Can you work these out from the model? Positions are in its coordinate system, mm. Face numbers are marked on the shaded views. Coordinates: 2 decimals unless noted, no trailing zeros. Order: outer loops, then holes, each group sorted by start corner. A loop starts at its lowest first (then second) coordinate and runs counter-clockwise, first axis right, second up. Notation, with made-up numbers: (8.5, 43.5) -> (31.5, 43.5) arc R8 cw to (31.5, 57.5) -> close; hole circle Ø9 at (62, -34.75). An arc over 180 degrees is marked (long way). Use a Markdown table: item, result. Add a question column.
1. We'd pull the mould along X, two halves only. Please class the marked faces 1 and 2: pulls with the +X half, pulls with the -X half, needs draft (parallel to the pull), parting line crosses it, or undercut.
2. Suppose I cut it at C-C, the plane z = 5.5. List the corners of the cut face in (x, y) for me.
3. Suppose I cut it at A-A, the plane y = 0. List the corners of the cut face in (x, z) for me.
4. If I drill on line 1 along Y through (x, z) = (-1.15, 4.5); line 2 along Y through (x, z) = (0.5, 1.25); line 3 along X through (y, z) = (-0.85, 2), over which ranges is the centre line in solid material (lowest first)? Write a range as from..to.
5. For pin 1 Ø1 at (x, z) = (-1.5, 3) entering from -Y; pin 2 Ø2.5 at (y, z) = (-0.5, 3.5) entering from -X; pin 3 Ø1.5 at (y, z) = (-1.5, 1.5) entering from +X, each with a flat end and sliding along its axis, tell me the tip position at first contact or that it passes through.
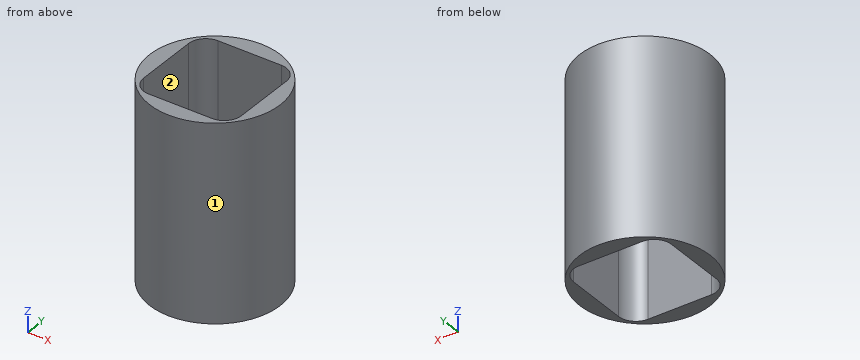
```python
from build123d import *

# Parameters (mm, degrees)
F0_R     = 2.1209
F1_DEPTH = 6.35
F3_DEPTH = 25.4


with BuildPart() as f1:
    # F0 (on Top) → F1 (new body)
    with BuildSketch(Plane.XY):
        Circle(F0_R)
    extrude(amount=F1_DEPTH)

    # F2 (on Top) → F3 (cut)
    with BuildSketch(Plane.XY):
        with BuildLine():
            Line((1.0287, 1.5875), (-1.0287, 1.5875))
            ThreePointArc((-1.0287, 1.5875), (-1.423831, 1.423831), (-1.5875, 1.0287))
            Line((-1.5875, 1.0287), (-1.5875, -1.0287))
            ThreePointArc((-1.5875, -1.0287), (-1.423831, -1.423831), (-1.0287, -1.5875))
            Line((-1.0287, -1.5875), (1.0287, -1.5875))
            ThreePointArc((1.0287, -1.5875), (1.423831, -1.423831), (1.5875, -1.0287))
            Line((1.5875, -1.0287), (1.5875, 1.0287))
            ThreePointArc((1.5875, 1.0287), (1.423831, 1.423831), (1.0287, 1.5875))
        make_face()
    extrude(amount=F3_DEPTH, mode=Mode.SUBTRACT)


solid = f1.part
```
Worked out:
| question | item | result |
|---|---|---|
| 1 | face 1 | parting line crosses it |
| 1 | face 2 | undercut |
| 2 | outline | circle Ø4.24 at (0, 0); hole (-1.59, -1.03) arc R0.56 ccw to (-1.03, -1.59) -> (1.03, -1.59) arc R0.56 ccw to (1.59, -1.03) -> (1.59, 1.03) arc R0.56 ccw to (1.03, 1.59) -> (-1.03, 1.59) arc R0.56 ccw to (-1.59, 1.03) -> close |
| 3 | outline | (-2.12, 0) -> (-1.59, 0) -> (-1.59, 6.35) -> (-2.12, 6.35) -> close; (1.59, 0) -> (2.12, 0) -> (2.12, 6.35) -> (1.59, 6.35) -> close |
| 4 | line 1 | y = -1.78..-1.57, 1.57..1.78 |
| 4 | line 2 | y = -2.06..-1.59, 1.59..2.06 |
| 4 | line 3 | x = -1.94..-1.59, 1.59..1.94 |
| 5 | pin 1 | stops at y = -1.87 |
| 5 | pin 2 | stops at x = -2.12 |
| 5 | pin 3 | stops at x = 1.98 |
